```python
from build123d import *

# Parameters (mm, degrees)
SKETCH_1_W          = 80
SKETCH_1_H          = 40
EXTRUDE_2_DEPTH     = 10
SKETCH_4_W          = 10
SKETCH_4_H          = 40
EXTRUDE_3_DEPTH     = 50
SKETCH_5_R          = 2.5
CUT_EXTRUDE_2_DEPTH = 93.736184955
SKETCH_6_W          = 130
SKETCH_6_H          = 10
EXTRUDE_4_DEPTH     = 30
SKETCH_7_W          = 130
SKETCH_7_H          = 10
EXTRUDE_5_DEPTH     = 30
SKETCH_8_R          = 2.5
CUT_EXTRUDE_3_DEPTH = 104.440804328
SKETCH_10_R         = 2.5
CUT_EXTRUDE_4_DEPTH = 104.440804328


with BuildPart() as part:
    # 草图1 → 凸台-拉伸2 (new body)
    with BuildSketch(Plane.XY):
        Rectangle(SKETCH_1_W, SKETCH_1_H)
    extrude(amount=EXTRUDE_2_DEPTH)

    # 草图4 → 凸台-拉伸3 (add)
    with BuildSketch(Plane.ZY.offset(40)):
        with Locations((5, 0)):
            Rectangle(SKETCH_4_W, SKETCH_4_H)
    extrude(amount=EXTRUDE_3_DEPTH)

    # 草图5 → 切除-拉伸2 (cut, through all)
    with BuildSketch(Plane.XY.offset(10)):
        with Locations((-85, 0)):
            Circle(SKETCH_5_R)
    extrude(amount=-CUT_EXTRUDE_2_DEPTH, mode=Mode.SUBTRACT)

    # 草图6 → 凸台-拉伸4 (add)
    with BuildSketch(Plane.XZ.offset(20)):
        with Locations((-25, 5)):
            Rectangle(SKETCH_6_W, SKETCH_6_H)
    extrude(amount=EXTRUDE_4_DEPTH)

    # 草图7 → 凸台-拉伸5 (add)
    with BuildSketch(Plane(origin=(0, 20, 0), x_dir=(1, 0, 0), z_dir=(0, 1, 0))):
        with Locations((-25, -5)):
            Rectangle(SKETCH_7_W, SKETCH_7_H)
    extrude(amount=EXTRUDE_5_DEPTH)

    # 草图8 → 切除-拉伸3 (cut, through all)
    with BuildSketch(Plane.XY.offset(10)):
        with Locations((35, -45)):
            Circle(SKETCH_8_R)
        with Locations(Location((35, 45, 0), (0, 0, 180))):
            Circle(SKETCH_8_R)
    extrude(amount=-CUT_EXTRUDE_3_DEPTH, mode=Mode.SUBTRACT)

    # 草图10 → 切除-拉伸4 (cut, through all)
    with BuildSketch(Plane.XY.offset(10)):
        with Locations((-85, 40)):
            Circle(SKETCH_10_R)
        with Locations((-85, -40)):
            Circle(SKETCH_10_R)
    extrude(amount=-CUT_EXTRUDE_4_DEPTH, mode=Mode.SUBTRACT)


solid = part.part
```
Verification items for the finished model (mm, model axes). Coordinates: 2 decimals unless noted, no trailing zeros. Order: outer loops, then holes, each group sorted by start corner. A loop starts at its lowest first (then second) coordinate and runs counter-clockwise, first axis right, second up. Notation, with made-up numbers: (-4.75, -39) -> (40.25, -39) arc R15 cw to (40.25, -15) -> close; hole circle Ø3 at (-5, -17). An arc over 180 degrees is marked (long way). Put each result on its own line as item: value. Start each with the question number.
1) Material ranges on L1, parallel to Y at x = -85, z = 6.75; L2, parallel to Y at x = 35, z = 4.25; L3, parallel to X at y = 44, z = 1.75, recorded low to high.
2) Cross-section at B-B (x = 35). Enter the section's corners in (y, z), plus the area to 3 significant figures.
3) Cross-section at A-A (x = -85). Enter the section's corners in (y, z).
4) Cross-section at C-C (y = 0). Enter the section's corners in (x, z).
5) Release check for a two-part mould opening along Y. For faces 1 (the flat face through (-26, -1, 10)), 2 (the cylindrical face through (-87, -41.5, 5.1)), 3 (the flat face through (-26, 50, 5)) record: pulls with the +Y half, pulls with the -Y half, needs draft (parallel to the pull), parting line crosses it, or undercut.
Geometry check:
1. L1: y = -50 to -42.5, -37.5 to -2.5, 2.5 to 37.5, 42.5 to 50
1. L2: y = -50 to -47.5, -42.5 to 42.5, 47.5 to 50
1. L3: x = -90 to 32.71, 37.29 to 40
2. outline: (-50, 0) -> (-47.5, 0) -> (-47.5, 10) -> (-50, 10) -> close; (-42.5, 0) -> (42.5, 0) -> (42.5, 10) -> (-42.5, 10) -> close; (47.5, 0) -> (50, 0) -> (50, 10) -> (47.5, 10) -> close
2. area: 900 mm^2
3. outline: (-50, 0) -> (-42.5, 0) -> (-42.5, 10) -> (-50, 10) -> close; (-37.5, 0) -> (-2.5, 0) -> (-2.5, 10) -> (-37.5, 10) -> close; (2.5, 0) -> (37.5, 0) -> (37.5, 10) -> (2.5, 10) -> close; (42.5, 0) -> (50, 0) -> (50, 10) -> (42.5, 10) -> close
4. outline: (-90, 0) -> (-87.5, 0) -> (-87.5, 10) -> (-90, 10) -> close; (-82.5, 0) -> (40, 0) -> (40, 10) -> (-82.5, 10) -> close
5. face 1: needs draft
5. face 2: undercut
5. face 3: pulls with the +Y half
